```python
from build123d import *

# Parameters (mm, degrees)
BOSS_EXTRUDE1_DEPTH = 6.1


with BuildPart() as part:
    # Sketch2 → Boss-Extrude1 (new, symmetric)
    with BuildSketch(Plane(origin=(0, 0, 0), x_dir=(0, 0, -1), z_dir=(1, 0, 0))):
        with BuildLine():
            Line((2.015254326, 2.015254326), (8.724964183, 8.724964183))
            ThreePointArc((8.724964183, 8.724964183), (10.299695568, 9.304298721), (11.761446185, 8.48047072))
            ThreePointArc((11.761446185, 8.48047072), (13.798387038, 4.455840567), (14.5, 0))
            Line((14.5, 0), (2.85, 0))
            ThreePointArc((2.85, 0), (1.090647782, -2.633056668), (-2.015254326, -2.015254326))
            Line((-2.015254326, -2.015254326), (-10.253048327, -10.253048327))
            ThreePointArc((-10.253048327, -10.253048327), (-12.907688125, -6.606177963), (-14.313196708, -2.32))
            ThreePointArc((-14.313196708, -2.32), (-13.8621173, -0.70385186), (-12.338962679, 0))
            Line((-12.338962679, 0), (-2.85, 0))
            ThreePointArc((-2.85, 0), (-1.090647782, 2.633056668), (2.015254326, 2.015254326))
        make_face()
    extrude(amount=BOSS_EXTRUDE1_DEPTH, both=True)


solid = part.part
```
Build history of the part. All positions in model axes, mm. A direction names the side the tool comes from. Round coordinates to 2 decimals unless told otherwise and drop trailing zeros. Write each loop counter-clockwise with the first axis right and the second up, starting at its lowest first coordinate (ties: lowest second). Pieces come first, ordered by that corner, then holes.
1) Drill centre lines: probe 1 along Z at (x, y) = (-0.5, -3.5); probe 2 along Z at (x, y) = (4.5, 3.5); probe 3 along Y at (x, z) = (4.75, 12). Where is each one in solid material? Low to high.
2) Band-saw the part on D-D, the plane y = -4.25. List the corners of the cut face in (x, z).
3) Band-saw the part on A-A, the plane y = 2.5. List the corners of the cut face in (x, z).
4) Pin check, flat tips, straight feed: pin 1 (2 mm diameter, centred on x = -0.5, y = -6.5, fed in from -Z); pin 2 (6 mm diameter, centred on x = -1.5, y = 2.5, fed in from +Z); pin 3 (2 mm diameter, centred on x = -2.5, z = 9, fed in from +Y). Stop position of each tip, or through.
5) 3-axis set-ups, long thin cutter, end or side, ignore diameter. For faces 4 (the cylindrical face through (0.085, 9.306, -10.276)), 5 (the flat face through (0, 0, -9)): which of +Z, -Z, +X, -X, +Y, -Y reach the whole face in a straight line?
6) Band-saw the part on B-B, the plane x = -5.25. List the corners of the cut face in (y, z), and give its area (3 significant figures).
7) Band-saw the part on C-C, the plane z = -4.5. List the corners of the cut face in (x, y).
8) Mould opens along Z. For faces 1 (the flat face through (0, 0, 8)), 2 (the cylindrical face through (0.085, 2.615, 1.134)), 3 (the cylindrical face through (0.09, -6.66, 12.88)) say: +Z half, -Z half, draft (parallel to the pull), parting line (faces both ways), or undercut.
Ans:
1. probe 1: z = 3.5 to 14.07
1. probe 2: z = -14.07 to -3.5
1. probe 3: y = -8.14 to 0
2. outline: (-6.1, 4.25) - (6.1, 4.25) - (6.1, 13.86) - (-6.1, 13.86) - close
3. outline: (-6.1, -14.28) - (6.1, -14.28) - (6.1, -2.5) - (-6.1, -2.5) - close; (-6.1, -1.37) - (6.1, -1.37) - (6.1, 1.37) - (-6.1, 1.37) - close
4. pin 1: stops at z = 5.5
4. pin 2: stops at z = 13.66
4. pin 3: stops at y = 0
5. face 4: +X, -X, +Y
5. face 5: -Z, +X, -X, -Y
6. outline: (-10.25, 10.25) - (-2.02, 2.02) arc R2.85 ccw to (0, -2.85) - (0, -14.5) arc R14.5 ccw to (8.48, -11.76) arc R2 ccw to (8.72, -8.72) - (2.02, -2.02) arc R2.85 ccw to (0, 2.85) - (0, 12.34) arc R2 ccw to (-2.32, 14.31) arc R14.5 ccw to start
6. area: 182 mm2
7. outline: (-6.1, 0) - (6.1, 0) - (6.1, 4.5) - (-6.1, 4.5) - close
8. face 1: draft
8. face 2: undercut
8. face 3: +Z half
